from build123d import *

# Parameters (mm, degrees)
CYLINDER070_R           = 2.5
CYLINDER070_DEPTH       = 2
CYLINDER069_R           = 1.5
CYLINDER069_DEPTH       = 10
BODY007_PLACEMENT_ANGLE = 90
ARRAY001039_Z_COUNT     = 5
ARRAY001039_Z_PITCH     = 20
BOX037_W                = 10
BOX037_H                = 2
BOX037_DEPTH            = 100


with BuildPart() as screw_cone_hole:
    # Cone005 → Cone005 (revolve)
    with BuildSketch(Plane.XZ):
        Polygon((0, 0), (2.5, 0), (1.8, 2), (0, 2), align=None)
    revolve(axis=Axis((0, 0, 0), (0, 0, 1)))


with BuildPart() as screw_head_hole:
    # Cylinder070 → Cylinder070 (new body)
    with BuildSketch(Plane.XY.offset(-2)):
        Circle(CYLINDER070_R)
    extrude(amount=CYLINDER070_DEPTH)


with BuildPart() as screw_hole_array:
    # Cylinder069 → Cylinder069 (new body)
    with BuildSketch(Plane.XY):
        Circle(CYLINDER069_R)
    extrude(amount=CYLINDER069_DEPTH)

    # Fusion047: union screw cone hole, screw head hole
    add(screw_cone_hole.part)
    add(screw_head_hole.part)


with BuildPart() as screw_hole_array_1:
    # Body007 placement: moved
    add(screw_hole_array.part.moved(Location((0, -4, 6))).rotate(Axis((0, -4, 6), (1, 0, 0)), BODY007_PLACEMENT_ANGLE))

    # Array001039 Z: screw hole array ×5


with BuildPart() as screw_hole_array_2:
    add(screw_hole_array_1.part)
    with Locations(*[(0, 0, i * ARRAY001039_Z_PITCH) for i in range(1, ARRAY001039_Z_COUNT)]):
        add(screw_hole_array_1.part)


with BuildPart() as wire_holder_cube_cut:
    # Box037 → Box037 (new body)
    with BuildSketch(Plane(origin=(-5, -6, -4), x_dir=(1, 0, 0), z_dir=(0, 0, 1))):
        with Locations((5, 1)):
            Rectangle(BOX037_W, BOX037_H)
    extrude(amount=BOX037_DEPTH)

    # Cut023010: cut screw hole array
    add(screw_hole_array_2.part, mode=Mode.SUBTRACT)


solid = wire_holder_cube_cut.part
Build history of the part. All positions in model axes, mm. Give positions to 0.01 mm unless a question says otherwise; leave off trailing zeros. Loops run counter-clockwise (first coordinate to the right, second up) from the corner with the lowest first, then second, coordinate; pieces in that order, holes last. Notation, with made-up numbers: (26, 43) - (73, 43) arc R22 cw to (73, 81) - close; hole circle Ø1 at (82, 20). An arc over 180 degrees is marked (long way). Write item = value, one per line. Start each with the question number.
1) Band-saw the part on A-A on y = -5.4. Give the cut face in (x, z), plus the area to 3 significant figures.
2) Band-saw the part on C-C on z = 6. Give the cut face in (x, y).
3) Pull direction X, two halves, no side cores. Call faces 1 (the flat face through (5, -5, 45)), 2 (the conical face through (-0.249, -5.681, 67.895)), 3 (the flat face through (0, -5, -4)): +X half, -X half, draft (parallel to the pull), parting line (faces both ways), or undercut.
4) Band-saw the part on B-B on x = 0. Give the cut face in (y, z).
5) Probe probe 1 along Z at (x, y) = (-0.5, -4.05); probe 2 along Z at (x, y) = (1.5, -5.4); probe 3 along X at (y, z) = (-5.1, 47). List the from-to ranges inside material, lowest first. Write a range as from..to.
Final values:
q1.outline = (-5, -4) - (5, -4) - (5, 96) - (-5, 96) - close; hole circle Ø4.02 at (0, 6); hole circle Ø4.02 at (0, 26); hole circle Ø4.02 at (0, 46); hole circle Ø4.02 at (0, 66); hole circle Ø4.02 at (0, 86)
q1.area = 937 mm²
q2.outline = (-5, -6) - (-1.8, -6) - (-2.5, -4) - (-5, -4) - close; (1.8, -6) - (5, -6) - (5, -4) - (2.5, -4) - close
q3.face_1 = +X half
q3.face_2 = undercut
q3.face_3 = draft
q4.outline = (-6, -4) - (-4, -4) - (-4, 3.5) - (-6, 4.2) - close; (-6, 7.8) - (-4, 8.5) - (-4, 23.5) - (-6, 24.2) - close; (-6, 27.8) - (-4, 28.5) - (-4, 43.5) - (-6, 44.2) - close; (-6, 47.8) - (-4, 48.5) - (-4, 63.5) - (-6, 64.2) - close; (-6, 67.8) - (-4, 68.5) - (-4, 83.5) - (-6, 84.2) - close; (-6, 87.8) - (-4, 88.5) - (-4, 96) - (-6, 96) - close
q5.probe_1 = -4..3.57, 8.43..23.57, 28.43..43.57, 48.43..63.57, 68.43..83.57, 88.43..96
q5.probe_2 = -4..4.66, 7.34..24.66, 27.34..44.66, 47.34..64.66, 67.34..84.66, 87.34..96
q5.probe_3 = -5..-1.86, 1.86..5
